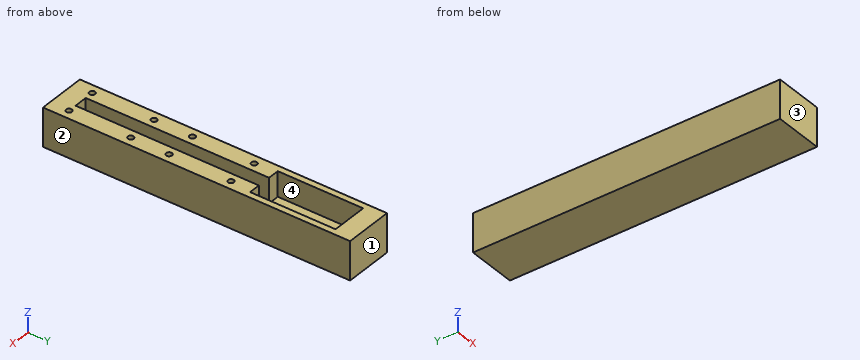
```python
from build123d import *

# Parameters (mm, degrees)
SKETCH_W        = 25.4
SKETCH_H        = 160
PAD_DEPTH       = 20
POCKET_DEPTH    = 13
SKETCH002_R     = 1.5
POCKET001_DEPTH = 10


with BuildPart() as part:
    # Sketch → Pad (new body)
    with BuildSketch(Plane.XY):
        with Locations((0, 80)):
            Rectangle(SKETCH_W, SKETCH_H)
    extrude(amount=PAD_DEPTH)

    # Sketch001 (on Face6 of Pad) → Pocket (cut)
    with BuildSketch(Plane.XY.offset(20)):
        Polygon((-9.5, 150), (9.5, 150), (9.5, 105.5), (3.5, 105.5), (3.5, 10), (-3.5, 10), (-3.5, 105.5), (-9.5, 105.5), align=None)
    extrude(amount=-POCKET_DEPTH, mode=Mode.SUBTRACT)

    # Sketch002 (on Face5 of Pocket) → Pocket001 (cut)
    with BuildSketch(Plane.XY.offset(20)):
        with Locations((-8, 94.4)):
            Circle(SKETCH002_R)
        with Locations((-8, 62.2)):
            Circle(SKETCH002_R)
        with Locations((8, 94.4)):
            Circle(SKETCH002_R)
        with Locations((8, 62.2)):
            Circle(SKETCH002_R)
        with Locations((-8, 42.2)):
            Circle(SKETCH002_R)
        with Locations((-8, 10)):
            Circle(SKETCH002_R)
        with Locations((8, 42.2)):
            Circle(SKETCH002_R)
        with Locations((8, 10)):
            Circle(SKETCH002_R)
    extrude(amount=-POCKET001_DEPTH, mode=Mode.SUBTRACT)


solid = part.part
```
CAD build for the part. Positions are in the model's coordinates, mm. Face numbers are marked on the shaded views. Round coordinates to 2 decimals unless told otherwise and drop trailing zeros. Order: outer loops, then holes, each group sorted by start corner. A loop starts at its lowest first (then second) coordinate and runs counter-clockwise, first axis right, second up. Notation, with made-up numbers: (36.5, 25.5) - (56.5, 25.5) arc R8 ccw to (56.5, 38.5) - close; hole circle Ø8 at (18, 84). An arc over 180 degrees is marked (long way). Use CSV: the item, a comma, the result in double quotes. Start each with the question number.
1) Pin check, flat tip, straight feed: pin 1 Ø0.9 at (x, y) = (8, 42) entering from +Z. Stop position of the tip, or through.
2) Two-plate mould, pull along Y, no slides. Class the marked faces 1, 2, 3 and 4: pulls with the +Y half, pulls with the -Y half, needs draft (parallel to the pull), parting line crosses it, or undercut.
3) Wall check: L1, parallel to X at y = 94.4, z = 17; L2, parallel to Y at x = 0.5, z = 9.5; L3, parallel to Y at x = 8, z = 15.5. Give the ranges that are in metal, low to high. Write a range as [from, to].
4) Saw through at A-A (z = 18). Count the separate pieces of the cut face and the enclosed holes in it, and give its area (3 significant figures).
5) Saw through at D-D (x = 2). List the corners of the cut face in (y, z).
6) Saw through at B-B (x = -8). List the corners of the cut face in (y, z), and give its area (3 significant figures).
7) Saw through at C-C (y = 42.2). List the corners of the cut face in (x, z).
Values follow:
1,pin 1,"stops at z = 10"
2,face 1,"pulls with the +Y half"
2,face 2,"needs draft"
2,face 3,"pulls with the -Y half"
2,face 4,"undercut"
3,L1,"x = [-12.7, -9.5], [-6.5, -3.5], [3.5, 6.5], [9.5, 12.7]"
3,L2,"y = [0, 10], [150, 160]"
3,L3,"y = [0, 8.5], [11.5, 40.7], [43.7, 60.7], [63.7, 92.9], [95.9, 105.5], [150, 160]"
4,separate pieces,"1"
4,enclosed holes,"9"
4,area,"2,490 mm2"
5,outline,"(0, 0) - (160, 0) - (160, 20) - (150, 20) - (150, 7) - (10, 7) - (10, 20) - (0, 20) - close"
6,outline,"(0, 0) - (160, 0) - (160, 20) - (150, 20) - (150, 7) - (105.5, 7) - (105.5, 20) - (95.9, 20) - (95.9, 10) - (92.9, 10) - (92.9, 20) - (63.7, 20) - (63.7, 10) - (60.7, 10) - (60.7, 20) - (43.7, 20) - (43.7, 10) - (40.7, 10) - (40.7, 20) - (11.5, 20) - (11.5, 10) - (8.5, 10) - (8.5, 20) - (0, 20) - close"
6,area,"2,500 mm2"
7,outline,"(-12.7, 0) - (12.7, 0) - (12.7, 20) - (9.5, 20) - (9.5, 10) - (6.5, 10) - (6.5, 20) - (3.5, 20) - (3.5, 7) - (-3.5, 7) - (-3.5, 20) - (-6.5, 20) - (-6.5, 10) - (-9.5, 10) - (-9.5, 20) - (-12.7, 20) - close"
